Geometry check sheet. Reference: the model listing, model coordinates, mm. A direction names the side the tool comes from. Coordinates: 2 decimals unless noted, no trailing zeros. Loops run counter-clockwise (first coordinate to the right, second up) from the corner with the lowest first, then second, coordinate; pieces in that order, holes last. Notation, with made-up numbers: (-7.5, 81.25) -> (13.5, 81.25) arc R30 ccw to (13.5, 106.25) -> close; hole circle Ø8 at (-8.5, 2.25). An arc over 180 degrees is marked (long way). Answer as a JSON object with one key per item and string values.
from build123d import *

# Parameters (mm, degrees)
EXTRUDE_1_DEPTH          = 3
SKETCH_2_R               = 1.525
CUT_EXTRUDE_1_DEPTH      = 4
SKETCH_3_R               = 1.275
CUT_EXTRUDE_2_DEPTH      = 4
SKETCH_5_W               = 6.5
SKETCH_5_H               = 95
CUT_EXTRUDE_4_DEPTH      = 4
FILLET_3_R               = 2
CUT_EXTRUDE_5_DEPTH      = 1
CUT_EXTRUDE_5_DEPTH_BACK = 4
FILLET_4_R               = 1
CUT_EXTRUDE_6_DEPTH      = 1
CUT_EXTRUDE_6_DEPTH_BACK = 4


with BuildPart() as part:
    # 草图1 → 凸台-拉伸1 (new body)
    with BuildSketch(Plane(origin=(0, 0, 0), x_dir=(1, 0, 0), z_dir=(0, 1, 0))):
        Polygon((33, -55), (33, 0), (33, 40), (-55, 40), (-55, -111), (0, -111), (0, -55), align=None)
    extrude(amount=EXTRUDE_1_DEPTH)

    # 草图2 → 切除-拉伸1 (cut, through all)
    with BuildSketch(Plane(origin=(0, 3, 0), x_dir=(1, 0, 0), z_dir=(0, 1, 0))):
        with Locations((-37.5, -107)):
            Circle(SKETCH_2_R)
        with Locations((-17.5, -107)):
            Circle(SKETCH_2_R)
        with Locations((-37.5, -75)):
            Circle(SKETCH_2_R)
        with Locations((-17.5, -75)):
            Circle(SKETCH_2_R)
        with Locations((-42, 36)):
            Circle(SKETCH_2_R)
        with Locations((-22, 36)):
            Circle(SKETCH_2_R)
        with Locations((-5.25, 36)):
            Circle(SKETCH_2_R)
        with Locations((14.75, 36)):
            Circle(SKETCH_2_R)
    extrude(amount=-CUT_EXTRUDE_1_DEPTH, mode=Mode.SUBTRACT)

    # 草图3 → 切除-拉伸2 (cut, through all)
    with BuildSketch(Plane(origin=(0, 3, 0), x_dir=(1, 0, 0), z_dir=(0, 1, 0))):
        with Locations((16.75, 20)):
            Circle(SKETCH_3_R)
        with Locations((-46.25, 20)):
            Circle(SKETCH_3_R)
        with Locations((16.75, -22)):
            Circle(SKETCH_3_R)
        with Locations((-46.25, -22)):
            Circle(SKETCH_3_R)
    extrude(amount=-CUT_EXTRUDE_2_DEPTH, mode=Mode.SUBTRACT)

    # 草图5 → 切除-拉伸4 (cut, through all)
    with BuildSketch(Plane(origin=(0, 3, 0), x_dir=(1, 0, 0), z_dir=(0, 1, 0))):
        with Locations((29.75, -7.5)):
            Rectangle(SKETCH_5_W, SKETCH_5_H)
    extrude(amount=-CUT_EXTRUDE_4_DEPTH, mode=Mode.SUBTRACT)

    # 圆角3
    fillet_3_edges = [part.edges().sort_by_distance(p)[0] for p in [
        (0, 1.5, 111),
        (-55, 1.5, 111),
        (-55, 1.5, -40),
        (0, 1.5, 55),
        (26.5, 1.5, 55),
        (26.5, 1.5, -40),
    ]]
    fillet(fillet_3_edges, radius=FILLET_3_R)

    # 草图6 → 切除-拉伸5 (cut, two sides)
    with BuildSketch(Plane(origin=(0, 3, 0), x_dir=(1, 0, 0), z_dir=(0, 1, 0))) as cut_extrude_5_sk:
        Polygon((-36.75, 29), (8.25, 29), (-14.25, -4.5), align=None)
        Polygon((-36.75, 18.238752654), (-36.75, -33.238752654), (-19.462778068, -7.5), align=None)
        Polygon((-9.037221932, -7.5), (8.25, 18.238752654), (8.25, -33.238752654), align=None)
        Polygon((-36.75, -44), (8.25, -44), (-14.25, -10.5), align=None)
    extrude(amount=CUT_EXTRUDE_5_DEPTH, mode=Mode.SUBTRACT)
    extrude(cut_extrude_5_sk.sketch, amount=-CUT_EXTRUDE_5_DEPTH_BACK, mode=Mode.SUBTRACT)

    # 圆角4
    fillet_4_edges = [part.edges().sort_by_distance(p)[0] for p in [
        (-36.75, 1.5, -18.238752654),
        (-19.462778068, 1.5, 7.5),
        (-36.75, 1.5, 33.238752654),
        (8.25, 1.5, 33.238752654),
        (-9.037221932, 1.5, 7.5),
        (8.25, 1.5, -18.238752654),
        (-36.75, 1.5, 44),
        (-14.25, 1.5, 10.5),
        (8.25, 1.5, 44),
        (-14.25, 1.5, 4.5),
        (-36.75, 1.5, -29),
        (8.25, 1.5, -29),
    ]]
    fillet(fillet_4_edges, radius=FILLET_4_R)

    # 草图7 → 切除-拉伸6 (cut, two sides)
    with BuildSketch(Plane(origin=(0, 3, 0), x_dir=(1, 0, 0), z_dir=(0, 1, 0))) as cut_extrude_6_sk:
        with BuildLine():
            Line((-37.5, -52), (-17.5, -52))
            ThreePointArc((-17.5, -52), (-8.5, -61), (-17.5, -70))
            Line((-17.5, -70), (-37.5, -70))
            ThreePointArc((-37.5, -70), (-46.5, -61), (-37.5, -52))
        make_face()
        with BuildLine():
            Line((-37.5, -82), (-17.5, -82))
            ThreePointArc((-17.5, -82), (-8.5, -91), (-17.5, -100))
            Line((-17.5, -100), (-37.5, -100))
            ThreePointArc((-37.5, -100), (-46.5, -91), (-37.5, -82))
        make_face()
    extrude(amount=CUT_EXTRUDE_6_DEPTH, mode=Mode.SUBTRACT)
    extrude(cut_extrude_6_sk.sketch, amount=-CUT_EXTRUDE_6_DEPTH_BACK, mode=Mode.SUBTRACT)


solid = part.part
1. Section check A-A, the plane z = 107. Record the boundary of the cut face in (x, y) (3 decimals).
Evaluation:
{"outline": "(-55, 0) -> (-39.025, 0) -> (-39.025, 3) -> (-55, 3) -> close; (-35.975, 0) -> (-19.025, 0) -> (-19.025, 3) -> (-35.975, 3) -> close; (-15.975, 0) -> (0, 0) -> (0, 3) -> (-15.975, 3) -> close"}
2. Tool access check on faces 4 (the face through (-27, 2, 100)), 5 (the face through (-24, 3, 18)), 6 (the face through (0, 1, 83)). Record the directions out of +Z, -Z, +X, -X, +Y, -Y that give a thin tool (end or side, any length) a straight path to the whole face; none if there is none.
Evaluation:
{"face 4": "+Y, -Y", "face 5": "+Z, -Z, +X, -X, +Y", "face 6": "+Z, +X, +Y, -Y"}
3. Mould release check, pull along Z, two halves, no side actions. Record for faces 1 (the face through (-55, 1, 34)), 2 (the face through (-14, 1, -40)), 3 (the face through (-8.502, 1.521, 90.802)): released by +Z, released by -Z, zero draft, split by the parting line, or undercut.
Evaluation:
{"face 1": "zero draft", "face 2": "released by -Z", "face 3": "undercut"}
4. Depth check by flat-ended pin: P1, Ø3, axis at x = -46.25, z = -20, coming from the +Y side; P2, Ø1.8, axis at x = -17.5, z = 107, coming from the -Y side. Enter the tip coordinate at first touch or a pass-through.
Evaluation:
{"P1": "stops at y = 3", "P2": "passes through"}
5. Section check D-D, the plane y = 1.6. State how many separate pieces and enclosed holes the cut face has, then the cut area to 3 significant figures.
Evaluation:
{"separate pieces": "1", "enclosed holes": "18", "area": "7,130 mm^2"}
6. Thickness scan on probe 1 along X at (y, z) = (1.4, -36) (3 decimals); probe 2 along X at (y, z) = (1.5, 75) (3 decimals); probe 3 along Z at (x, y) = (16.75, 2.05) (3 decimals). Record the ranges inside material, lowest first. Write a range as from..to.
Evaluation:
{"probe 1": "x = -55..-43.525, -40.475..-23.525, -20.475..-6.775, -3.725..13.225, 16.275..26.5", "probe 2": "x = -55..-39.025, -35.975..-19.025, -15.975..0", "probe 3": "z = -40..-21.275, -18.725..20.725, 23.275..55"}
7. Section check C-C, the plane z = 91. Record the boundary of the cut face in (x, y), then the cut area to 3 significant figures.
Evaluation:
{"outline": "(-55, 0) -> (-46.5, 0) -> (-46.5, 3) -> (-55, 3) -> close; (-8.5, 0) -> (0, 0) -> (0, 3) -> (-8.5, 3) -> close", "area": "51.0 mm^2"}
8. Section check B-B, the plane x = -42. Record the boundary of the cut face in (y, z) (3 decimals), then the cut area to 3 significant figures.
Evaluation:
{"outline": "(0, -40) -> (3, -40) -> (3, -37.525) -> (0, -37.525) -> close; (0, -34.475) -> (3, -34.475) -> (3, 53.206) -> (0, 53.206) -> close; (0, 68.794) -> (3, 68.794) -> (3, 83.206) -> (0, 83.206) -> close; (0, 98.794) -> (3, 98.794) -> (3, 111) -> (0, 111) -> close", "area": "350 mm^2"}
